Can you work these out from the model? Positions are in its coordinate system, mm. A direction names the side the tool comes from. Give positions to 0.01 mm unless a question says otherwise; leave off trailing zeros. Order: outer loops, then holes, each group sorted by start corner. A loop starts at its lowest first (then second) coordinate and runs counter-clockwise, first axis right, second up. Notation, with made-up numbers: (20.5, -35) -> (54.5, -35) arc R24 cw to (54.5, -6) -> close; hole circle Ø6 at (43.5, -5.75). An arc over 180 degrees is marked (long way). Answer as CSV lines item,"result".
```python
from build123d import *

# Parameters (mm, degrees)
F0_W      = 2000
F0_H      = 2000
F1_DEPTH  = 200
F2_W      = 300
F2_H      = 300
F3_DEPTH  = 25
F5_D      = 25
F5_DEPTH  = 25
F5_TIP    = 7.5107577378
F6_D      = 150
F6_DEPTH  = 25
F6_TIP    = 45.0645464271
F7_W      = 182
F7_H      = 182
F8_DEPTH  = 300
F9_W      = 300
F9_H      = 300
F10_DEPTH = 25
F12_D     = 150
F12_DEPTH = 25
F12_TIP   = 45.0645464271


with BuildPart() as f1:
    # F0 (on Top) → F1 (new body)
    with BuildSketch(Plane.XY):
        with Locations((-3.9364807308, 344.8101401439)):
            Rectangle(F0_W, F0_H)
    extrude(amount=F1_DEPTH)

    # F2 (on face) → F3 (join)
    with BuildSketch(Plane.XY.offset(200)):
        with Locations((-3.9364807308, -220.0311138496)):
            Rectangle(F2_W, F2_H)
    extrude(amount=F3_DEPTH)

    # F5
    with Locations(Plane.XY.offset(225)):
        with Locations((-123.9364807308, -100.0311138496), (-123.9364807308, -340.0311138496), (116.0635192692, -340.0311138496), (116.0635192692, -100.0311138496)):
            Hole(F5_D / 2, depth=F5_DEPTH)
            with Locations((0, 0, -(F5_DEPTH + F5_TIP / 2))):  # 118° drill point
                Cone(0, F5_D / 2, F5_TIP, mode=Mode.SUBTRACT)

    # F6
    with Locations(Plane.XY.offset(225)):
        with Locations((-3.9364807308, -220.0311138496)):
            Hole(F6_D / 2, depth=F6_DEPTH)
            with Locations((0, 0, -(F6_DEPTH + F6_TIP / 2))):  # 118° drill point
                Cone(0, F6_D / 2, F6_TIP, mode=Mode.SUBTRACT)

    # F7 (on face) → F8 (join)
    with BuildSketch(Plane.XY.offset(225)):
        with BuildLine():
            Line((91.0635192692, -120.0311138496), (-98.9364807308, -120.0311138496))
            ThreePointArc((-98.9364807308, -120.0311138496), (-102.4720146367, -121.4955799437), (-103.9364807308, -125.0311138496))
            Line((-103.9364807308, -125.0311138496), (-103.9364807308, -315.0311138496))
            ThreePointArc((-103.9364807308, -315.0311138496), (-102.4720146367, -318.5666477555), (-98.9364807308, -320.0311138496))
            Line((-98.9364807308, -320.0311138496), (91.0635192692, -320.0311138496))
            ThreePointArc((91.0635192692, -320.0311138496), (94.5990531752, -318.5666477555), (96.0635192692, -315.0311138496))
            Line((96.0635192692, -315.0311138496), (96.0635192692, -125.0311138496))
            ThreePointArc((96.0635192692, -125.0311138496), (94.5990531752, -121.4955799437), (91.0635192692, -120.0311138496))
        make_face()
        with Locations((-3.9364807308, -220.0311138496)):
            Rectangle(F7_W, F7_H, mode=Mode.SUBTRACT)
    extrude(amount=F8_DEPTH)

    # F9 (on face) → F10 (join)
    with BuildSketch(Plane.XY.offset(525)):
        with Locations((-3.9364807308, -220.0311138496)):
            Rectangle(F9_W, F9_H)
    extrude(amount=F10_DEPTH)

    # F12
    with Locations(Plane.XY.offset(550)):
        with Locations((-3.9364807308, -220.0311138496)):
            Hole(F12_D / 2, depth=F12_DEPTH)
            with Locations((0, 0, -(F12_DEPTH + F12_TIP / 2))):  # 118° drill point
                Cone(0, F12_D / 2, F12_TIP, mode=Mode.SUBTRACT)


solid = f1.part
```
Item 1: Imagine slicing it at A-A, the plane z = 294.5. Please give me the cut outline in (x, y), then the cut area to 3 significant figures.
Numbers:
outline,"(-103.94, -315.03) arc R5 ccw to (-98.94, -320.03) -> (91.06, -320.03) arc R5 ccw to (96.06, -315.03) -> (96.06, -125.03) arc R5 ccw to (91.06, -120.03) -> (-98.94, -120.03) arc R5 ccw to (-103.94, -125.03) -> close; hole (-94.94, -311.03) -> (87.06, -311.03) -> (87.06, -129.03) -> (-94.94, -129.03) -> close"
area,"6,850 mm²"
Item 2: For faces 4 (the flat face through (-5, -320.031, 373)), 5 (the flat face through (-103.936, -219, 373)), 6 (the flat face through (-5, -129.031, 373)), which set-ups out of +Z, -Z, +X, -X, +Y, -Y let a thin tool reach every point of the face, with its end or its side?
Numbers:
face 4,"+X, -X, -Y"
face 5,"-X, +Y, -Y"
face 6,"none"
Item 3: Imagine slicing it at C-C, the plane x = -261.5. Please give me the cut outline in (y, z), then the cut area to 3 significant figures.
Numbers:
outline,"(-655.19, 0) -> (1344.81, 0) -> (1344.81, 200) -> (-655.19, 200) -> close"
area,"400,000 mm²"
Item 4: Imagine slicing it at B-B, the plane y = 894. Please give me the cut outline in (x, z), then the cut area to 3 significant figures.
Numbers:
outline,"(-1003.94, 0) -> (996.06, 0) -> (996.06, 200) -> (-1003.94, 200) -> close"
area,"400,000 mm²"
Item 5: For pin 1 (7.5 mm diameter, centred on x = -66.5, z = 218, fed in from +Y); pin 2 (1 mm diameter, centred on y = -265, z = 347.5, fed in from -X); pin 3 (3 mm diameter, centred on x = -242.5, y = -382.5, fed in from -Z); pin 4 (5 mm diameter, centred on x = -19.5, y = 411, fed in from +Z), each with a flat end and sliding along its axis, tell me the tip position at first contact or that it passes through.
Numbers:
pin 1,"stops at y = -70.03"
pin 2,"stops at x = -103.94"
pin 3,"stops at z = 0"
pin 4,"stops at z = 200"
Item 6: We'd pull the mould along X, two halves only. Please class faces 1 (the flat face through (996.064, 331, 99)), 2 (the flat face through (-86, -219, 525)), 3 (the flat face through (-73, -185, 550)): released by +X, released by -X, zero draft, split by the parting line, or undercut.
Numbers:
face 1,"released by +X"
face 2,"undercut"
face 3,"zero draft"
Item 7: Please list where these lines run through material, in increasing order: line 1 along Y through (x, z) = (7, 372); line 2 along Z through (x, y) = (600, -452).
Numbers:
line 1,"y = -320.03 to -311.03, -129.03 to -120.03"
line 2,"z = 0 to 200"
